For this review, take the finished solid that the model builds, in its own axes (mm). A direction names the side the tool comes from. Round coordinates to 2 decimals unless told otherwise and drop trailing zeros. Write each loop counter-clockwise with the first axis right and the second up, starting at its lowest first coordinate (ties: lowest second). Pieces come first, ordered by that corner, then holes. Notation, with made-up numbers: (21, 66) -> (68, 66) arc R23 ccw to (68, 86) -> close; hole circle Ø9 at (-36.5, 70.25). An arc over 180 degrees is marked (long way). Answer as CSV lines item,"result". Start each with the question number.
Item 1: Take a section at B-B on x = 0. Give the boundary of the cut face in (y, z).
Item 2: Take a section at C-C on z = -3.5. Give the boundary of the cut face in (x, y), then the cut area to 3 significant figures.
Item 3: Wall thickness on probe 1 along Z at (x, y) = (0, 4.25); probe 2 along Z at (x, y) = (0, 10.2); probe 3 along Y at (x, z) = (0, -3.3): over which ranges is each line inside the solid? List them lowest first. Write a range as from..to.
Item 4: Take a section at A-A on z = 0. Give the boundary of the cut face in (x, y), then the cut area to 3 significant figures.
Item 5: For pin 1 Ø1.5 at (x, y) = (-2, 2.5) entering from +Z; pin 2 Ø1 at (y, z) = (8.5, 1) entering from -X; pin 3 Ø3 at (y, z) = (4, -0.5) entering from +X, all flat-tipped, find the tip position at first contact; note any pin that passes through.
Item 6: Mouldability with a two-part tool opening along X and no side actions: class faces 1 (the flat face through (4, 12, -2)), 2 (the cylindrical face through (2.183, 6.93, 5.265)), 3 (the flat face through (2, 8.9, -2)) as +X half, -X half, draft (parallel to the pull), parting line (faces both ways), or undercut.
Item 7: Machinability: for faces 4 (the flat face through (0, 2, 6)), 5 (the cylindrical face through (0, 8, -4)), 6 (the flat face through (-2, 0, -2)), which of the approach directions +Z, -Z, +X, -X, +Y, -Y give a long, thin tool a straight path to every point of the face, cutting with its end or side? Answer none if there is none.
Item 8: Take a section at D-D on y = 5. Give the boundary of the cut face in (x, z), then the cut area to 3 significant figures.
```python
from build123d import *

# Parameters (mm, degrees)
F4_D     = 2
F4_DEPTH = 6.401


with BuildPart() as f2:
    # F1 (on Right) → F2 (revolve)
    with BuildSketch(Plane.YZ):
        Polygon((0, 2.1), (8.9, 2.1), (8.9, 4.05), (12, 4.05), (12, 5.7), (2, 5.7), (2, 6.4), (0, 6.4), align=None)
    revolve(axis=Axis((0, 5.7350749573, 0), (0, -1, 0)))

    # F4 (through all, one way)
    with BuildSketch(Plane.XY):
        with Locations((0, 7)):
            Circle(F4_D / 2)
    extrude(amount=-F4_DEPTH, mode=Mode.SUBTRACT)


solid = f2.part
```
Output values:
1,outline,"(0, -6.4) -> (2, -6.4) -> (2, -5.7) -> (6, -5.7) -> (6, -2.1) -> (0, -2.1) -> close; (0, 2.1) -> (8.9, 2.1) -> (8.9, 4.05) -> (12, 4.05) -> (12, 5.7) -> (2, 5.7) -> (2, 6.4) -> (0, 6.4) -> close; (8, -5.7) -> (12, -5.7) -> (12, -4.05) -> (8.9, -4.05) -> (8.9, -2.1) -> (8, -2.1) -> close"
2,outline,"(-5.36, 0) -> (5.36, 0) -> (5.36, 2) -> (4.5, 2) -> (4.5, 12) -> (2.04, 12) -> (2.04, 8.9) -> (-2.04, 8.9) -> (-2.04, 12) -> (-4.5, 12) -> (-4.5, 2) -> (-5.36, 2) -> close; hole circle Ø2 at (0, 7)"
2,area,"95.6 mm^2"
3,probe 1,"z = -5.7..-2.1, 2.1..5.7"
3,probe 2,"z = -5.7..-4.05, 4.05..5.7"
3,probe 3,"y = 0..6, 8..8.9"
4,outline,"(-6.4, 0) -> (-2.1, 0) -> (-2.1, 8.9) -> (-4.05, 8.9) -> (-4.05, 12) -> (-5.7, 12) -> (-5.7, 2) -> (-6.4, 2) -> close; (2.1, 0) -> (6.4, 0) -> (6.4, 2) -> (5.7, 2) -> (5.7, 12) -> (4.05, 12) -> (4.05, 8.9) -> (2.1, 8.9) -> close"
4,area,"77.1 mm^2"
5,pin 1,"stops at z = 6.24"
5,pin 2,"stops at x = -5.68"
5,pin 3,"stops at x = 5.7"
6,face 1,"draft"
6,face 2,"parting line"
6,face 3,"undercut"
7,face 4,"+Y"
7,face 5,"-Z"
7,face 6,"+Z, -Z, +X, -X, -Y"
8,outline,"circle Ø11.4 at (0, 0); hole circle Ø4.2 at (0, 0)"
8,area,"88.2 mm^2"
